Here's how the part is built. I have some questions about the finished solid (model axes, mm). A direction names the side the tool comes from. Round coordinates to 2 decimals unless told otherwise and drop trailing zeros. Order: outer loops, then holes, each group sorted by start corner. A loop starts at its lowest first (then second) coordinate and runs counter-clockwise, first axis right, second up. Notation, with made-up numbers: (86, 16.5) - (99, 16.5) arc R33 ccw to (99, 46.5) - close; hole circle Ø6 at (75.5, 62.5). An arc over 180 degrees is marked (long way). Answer as a JSON object with one key per item and string values.
Autodesk Inventor part; units mm, degrees
ref_plane "YZ Plane" through (0, 0, 0) normal (1, 0, 0) x (0, 1, 0)
ref_plane "XZ Plane" through (0, 0, 0) normal (0, 1, 0) x (-1, 0, 0)
ref_plane "XY Plane" through (0, 0, 0) normal (0, 0, 1) x (1, 0, 0)
ref_plane "Work Plane1" through (46.4934, 164.1502, -100.8153) normal (0, -0.1396054, 0.9902072) x (1, 0, 0)
sketch "Sketch1" plane through (46.4934, 164.1502, -100.8153) normal (0, -0.1396054, 0.9902072) x (1, 0, 0)
  circle A0 centre (-77.9553, -107.0952) radius 4.3235
  circle A1 centre (-77.9553, -107.0952) radius 4.1018
  point P0 (-46.4934, -148.4684)
extrude "Extrusion1" add sketch "Sketch1" against normal blind 25.4 contours A1
thread "Thread1"
sketch "Sketch2" plane through (46.4934, 164.1502, -100.8153) normal (0, -0.1396054, 0.9902072) x (1, 0, 0)
  circle A0 centre (-77.9553, -107.0952) radius 4.3235 construction
  line L0 (0, -50.1427) -> (0, 0) construction
  arc A1 (-38.2285, -91.2202) -> (0, -50.1427) centre (-77.9553, -15.9215) ccw construction
  line L1 (-38.2285, -91.2202) -> (-117.6821, -91.2202) construction
  arc A2 (-155.9106, -50.1427) -> (-117.6821, -91.2202) centre (-77.9553, -15.9215) ccw construction
  line L2 (-155.9106, -50.1427) -> (-155.9106, 0) construction
  line L3 (-155.9106, 0) -> (-159.0856, 0) construction
  line L4 (-159.0856, -50.1427) -> (-159.0856, 0) construction
  arc A3 (-159.0856, -50.1427) -> (-117.8938, -94.3952) centre (-77.9553, -15.9215) ccw construction
  line L5 (-117.8938, -94.3952) -> (-103.6066, -94.3952) construction
  line L6 (-103.6066, -94.3952) -> (-103.6066, -119.7952) construction
  line L7 (-52.304, -119.7952) -> (-103.6066, -119.7952) construction
  line L8 (-52.304, -94.3952) -> (-52.304, -119.7952) construction
  line L9 (-52.304, -94.3952) -> (-38.0167, -94.3952) construction
  arc A4 (-38.0167, -94.3952) -> (3.175, -50.1427) centre (-77.9553, -15.9215) ccw construction
  line L10 (3.175, 0) -> (3.175, -50.1427) construction
  line L11 (0, 0) -> (3.175, 0) construction
  line L12 (-96.3354, -100.2936) -> (-59.5752, -100.2936)
  line L13 (-59.5752, -100.2936) -> (-59.5752, -113.8968)
  line L14 (-59.5752, -113.8968) -> (-96.3354, -113.8968)
  line L15 (-96.3354, -113.8968) -> (-96.3354, -100.2936)
  line L16 (-96.3354, -107.0952) -> (-59.5752, -107.0952) construction
  line L17 (-77.9553, -100.2936) -> (-77.9553, -113.8968) construction
  point P0 (-46.4934, -148.4684)
extrude "Extrusion2" add sketch "Sketch2" along normal blind 6.35
sketch "Sketch4" plane through (-49.842, 51.3688, -116.7159) normal (0, -0.9902072, -0.1396054) x (1, 0, 0)
  line L0 (0, 0) -> (36.7602, 0) construction
  line L1 (36.7602, 0) -> (36.7602, 6.35) construction
  line L2 (0, 6.35) -> (36.7602, 6.35) construction
  line L3 (0, 0) -> (0, 6.35) construction
  line L4 (0, 15.2304) -> (36.7602, 15.2304) construction
  line L5 (36.7602, 21.5804) -> (0, 21.5804) construction
  line L6 (0, 21.5804) -> (0, 15.2304) construction
  line L7 (30.4102, 59.9083) -> (30.4102, 21.5804) construction
  line L8 (0, 30.4608) -> (30.4102, 30.4608) construction
  line L9 (0, 30.4608) -> (0, 36.8108) construction
  line L10 (6.35, 6.35) -> (6.35, 15.2304) construction
  line L11 (36.7602, 36.8108) -> (0, 36.8108) construction
  line L12 (0, 30.4608) -> (0, 36.8108) construction
  line L13 (36.7602, 15.2304) -> (36.7602, 36.8108) construction
  line L14 (0, 0) -> (0, 21.5804) construction
  line L15 (6.35, 6.35) -> (6.35, 15.2304)
  line L16 (6.35, 15.2304) -> (36.7602, 15.2304)
  line L17 (36.7602, 15.2304) -> (36.7602, 36.8108)
  line L18 (0, 36.8108) -> (36.7602, 36.8108)
  line L19 (0, 36.8108) -> (0, 30.4608)
  line L20 (0, 30.4608) -> (30.4102, 30.4608)
  line L21 (30.4102, 30.4608) -> (30.4102, 21.5804)
  line L22 (30.4102, 21.5804) -> (0, 21.5804)
  line L23 (0, 21.5804) -> (0, 6.35)
  line L24 (0, 6.35) -> (6.35, 6.35)
  line L25 (0, 6.35) -> (36.7602, 6.35)
  point P0 (49.842, 122.7443)
  dimension "d7" = 6.35
  dimension "d11" = 6.35
  dimension "d12" = 6.35
  dimension "d13" = 6.35
extrude "Extrusion3" add sketch "Sketch4" against normal up to surface (13.6032 mm away)
sketch "Sketch5" plane through (-49.842, 46.2298, -80.2656) normal (0, -0.1396054, 0.9902072) x (1, 0, 0)
  circle A0 centre (18.3801, 6.8016) radius 4.1018
  point P0 (49.842, -34.5716)
extrude "Extrusion4" cut sketch "Sketch5" against normal up to surface (6.35 mm away)
1. Imagine slicing it at C-C (x = -18). List the corners of the cut face in (y, z) for me, plus the area to 3 significant figures.
Responses:
{"outline": "(46.23, -80.27) - (49.24, -101.63) - (62.71, -99.74) - (59.7, -78.37) - close; (50.48, -110.43) - (51.37, -116.72) - (64.84, -114.82) - (63.95, -108.53) - close", "area": "380 mm2"}
2. If I drill on L1, parallel to Z at x = -42, y = 54.5; L2, parallel to Z at x = -36, y = 54.75; L3, parallel to Y at x = -33.5, z = -80.5, over which ranges is the centre line in solid material (lowest first)? Write a range as [from, to].
Responses:
{"L1": "[-116.27, -109.86], [-100.89, -94.48], [-85.51, -79.1]", "L2": "[-116.24, -109.83], [-100.86, -94.45], [-85.48, -79.06]", "L3": "[46.26, 49.54], [56.73, 60]"}
3. For P1, Ø4, axis at x = -45, y = 63, coming from the +Z side; P2, Ø5.5, axis at y = 56.5, z = -105, coming from the +X side, each with a flat end and sliding along its axis, tell me the tip position at first contact or that it passes through.
Responses:
{"P1": "z = -93.45", "P2": "x = -43.49"}
4. For faces 1 (the face through (-28.5, 55.88, -100.7)), 2 (the face through (-34.42, 55, -94.41)), 3 (the face through (-38.229, 53.757, -85.617)), 4 (the face through (-28.5, 57.312, -109.465)), which set-ups out of +Z, -Z, +X, -X, +Y, -Y let a thin tool reach every point of the face, with its end or its side?
Responses:
{"face 1": "+X, +Y", "face 2": "-X, -Y", "face 3": "-X, +Y", "face 4": "+X, -Y"}
5. Imagine slicing it at B-B (x = -37.5). List the corners of the cut face in (y, z) for me.
Responses:
{"outline": "(46.23, -80.27) - (47.12, -86.55) - (60.59, -84.65) - (59.7, -78.37) - close; (48.36, -95.35) - (49.24, -101.63) - (62.71, -99.74) - (61.83, -93.45) - close; (50.48, -110.43) - (51.37, -116.72) - (64.84, -114.82) - (63.95, -108.53) - close"}
6. Imagine slicing it at A-A (x = -33.5). List the corners of the cut face in (y, z) for me.
Responses:
{"outline": "(46.23, -80.27) - (47.12, -86.55) - (50.33, -86.1) - (49.44, -79.81) - close; (48.36, -95.35) - (49.24, -101.63) - (62.71, -99.74) - (61.83, -93.45) - close; (50.48, -110.43) - (51.37, -116.72) - (54.58, -116.26) - (58.12, -141.41) - (65.17, -140.42) - (61.63, -115.27) - (64.84, -114.82) - (63.95, -108.53) - close; (56.49, -78.82) - (57.38, -85.11) - (60.59, -84.65) - (59.7, -78.37) - close"}
7. Thinking about a two-plate mould opening in Z: for faces 5 (the face through (-27.55, 61.07, -127.99)), 6 (the face through (-49.842, 53, -82)), 7 (the face through (-27.55, 54.62, -82.24)), 8 (the face through (-35.8, 52.87, -79.33)), which applies, pulls with the +Z half, pulls with the -Z half, needs draft (parallel to the pull), parting line crosses it, or undercut?
Responses:
{"face 5": "undercut", "face 6": "needs draft", "face 7": "undercut", "face 8": "pulls with the +Z half"}
8. Imagine slicing it at D-D (z = -106). List the corners of the cut face in (x, y) for me.
Responses:
{"outline": "(-49.84, 49.86) - (-43.49, 49.86) - (-43.49, 63.6) - (-49.84, 63.6) - close"}
